```python
from build123d import *

# Parameters (mm, degrees)
F1_R      = 3
F5_DEPTH  = 7
F6_SIZE   = 2
F7_DEPTH  = 15.8
F1_R_2    = 5.35
F8_DEPTH  = 7
F9_SIZE   = 2
F1_R_3    = 7.5
F1_R_4    = 5.05
F10_DEPTH = 3
F1_R_5    = 3.15
F11_DEPTH = 10
F12_DEPTH = 1
F13_DEPTH = 4
F14_W     = 38.3726581931
F14_H     = 0.6922930479
F15_DEPTH = 1


with BuildPart() as f5:
    # F1 (on Top) → F5 (new body)
    with BuildSketch(Plane.XY):
        with BuildLine():
            Line((-67.5440824628, 59.7986807566), (-67.5440824628, 9.7986807566))
            Line((-67.5440824628, 9.7986807566), (-47.5440824628, 9.7986807566))
            Line((-47.5440824628, 9.7986807566), (-47.5440824628, 59.7986807566))
            ThreePointArc((-47.5440824628, 59.7986807566), (-57.5440824628, 69.7986807566), (-67.5440824628, 59.7986807566))
        make_face()
        with Locations((-57.5440824628, 59.7986807566)):
            Circle(F1_R, mode=Mode.SUBTRACT)
    extrude(amount=F5_DEPTH)

    # F6
    f6_edges = [f5.edges().sort_by_distance(p)[0] for p in [
        (-57.544082, 9.798681, 0),
        (-47.544082, 34.798681, 0),
        (-57.544082, 69.798681, 0),
        (-67.544082, 34.798681, 0),
    ]]
    chamfer(f6_edges, length=F6_SIZE)

    # F1 (on Top) → F7 (join)
    with BuildSketch(Plane.XY):
        with Locations((-57.5440824628, 59.7986807566)):
            Circle(F1_R)
    extrude(amount=F7_DEPTH)



with BuildPart() as f8:
    # F1 (on Top) → F8 (new body)
    with BuildSketch(Plane.XY):
        with BuildLine():
            ThreePointArc((-3.5915456533, 60.5911472063), (-13.5915456533, 70.5911472063), (-23.5915456533, 60.5911472063))
            Line((-23.5915456533, 60.5911472063), (-23.5915456533, 10.5911472063))
            Line((-23.5915456533, 10.5911472063), (-3.5915456533, 10.5911472063))
            Line((-3.5915456533, 10.5911472063), (-3.5915456533, 60.5911472063))
        make_face()
        with Locations((-13.5915456533, 60.5911472063)):
            Circle(F1_R_2, mode=Mode.SUBTRACT)
    extrude(amount=F8_DEPTH)

    # F9
    f9_edges = [f8.edges().sort_by_distance(p)[0] for p in [
        (-13.591546, 10.591147, 0),
        (-3.591546, 35.591147, 0),
        (-13.591546, 70.591147, 0),
        (-23.591546, 35.591147, 0),
    ]]
    chamfer(f9_edges, length=F9_SIZE)


with BuildPart() as f10:
    # F1 (on Top) → F10 (new body)
    with BuildSketch(Plane.XY):
        with Locations((-35.6929131355, 62.5116448375)):
            Circle(F1_R_3)
        with Locations((-35.6929131355, 62.5116448375)):
            Circle(F1_R_4, mode=Mode.SUBTRACT)
    extrude(amount=F10_DEPTH)

    # F1 (on Top) → F11 (join)
    with BuildSketch(Plane.XY):
        with Locations((-35.6929131355, 62.5116448375)):
            Circle(F1_R_4)
        with Locations((-35.6929131355, 62.5116448375)):
            Circle(F1_R_5, mode=Mode.SUBTRACT)
    extrude(amount=F11_DEPTH)

    # F1 (on Top) → F12 (join)
    with BuildSketch(Plane.XY):
        with Locations((-35.6929131355, 62.5116448375)):
            Circle(F1_R_5)
    extrude(amount=F12_DEPTH)


with BuildPart() as f13:
    # F1 (on Top) → F13 (new body)
    with BuildSketch(Plane.XY):
        with BuildLine():
            Line((-69.5440824628, 59.7986807566), (-69.5440824628, 7.7986807566))
            Line((-69.5440824628, 7.7986807566), (-45.5440824628, 7.7986807566))
            Line((-45.5440824628, 7.7986807566), (-45.5440824628, 59.7986807566))
            ThreePointArc((-45.5440824628, 59.7986807566), (-57.5440824628, 71.7986807566), (-69.5440824628, 59.7986807566))
        make_face()
        with BuildLine():
            ThreePointArc((-68.5440824628, 59.7986807566), (-57.5440824628, 70.7986807566), (-46.5440824628, 59.7986807566))
            Line((-46.5440824628, 59.7986807566), (-46.5440824628, 8.7986807566))
            Line((-46.5440824628, 8.7986807566), (-68.5440824628, 8.7986807566))
            Line((-68.5440824628, 8.7986807566), (-68.5440824628, 59.7986807566))
        make_face(mode=Mode.SUBTRACT)
    extrude(amount=F13_DEPTH)


with BuildPart() as f13b:
    # F1 (on Top) → F13, piece 2 (new body)
    with BuildSketch(Plane.XY):
        with BuildLine():
            Line((-25.5915456533, 60.5911472063), (-25.5915456533, 8.5911472063))
            Line((-25.5915456533, 8.5911472063), (-1.5915456533, 8.5911472063))
            Line((-1.5915456533, 8.5911472063), (-1.5915456533, 60.5911472063))
            ThreePointArc((-1.5915456533, 60.5911472063), (-13.5915456533, 72.5911472063), (-25.5915456533, 60.5911472063))
        make_face()
        with BuildLine():
            Line((-2.5915456533, 9.5911472063), (-24.5915456533, 9.5911472063))
            Line((-24.5915456533, 9.5911472063), (-24.5915456533, 60.5911472063))
            ThreePointArc((-24.5915456533, 60.5911472063), (-13.5915456533, 71.5911472063), (-2.5915456533, 60.5911472063))
            Line((-2.5915456533, 60.5911472063), (-2.5915456533, 9.5911472063))
        make_face(mode=Mode.SUBTRACT)
    extrude(amount=F13_DEPTH)


with BuildPart() as f5_1:
    add(f5.part)

    add(f8.part)  # F15 merges F8

    add(f10.part)  # F15 merges F10

    add(f13.part)  # F15 merges F13

    add(f13b.part)  # F15 merges F13b
    # F14 (on Top) → F15 (join)
    with BuildSketch(Plane.XY):
        with Locations((-36.1423902214, 55.9608265758)):
            Rectangle(F14_W, F14_H)
    extrude(amount=F15_DEPTH)


solid = f5_1.part
```
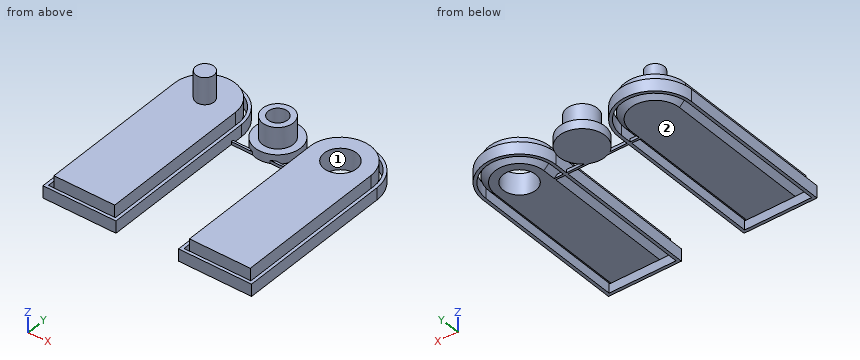
Here's how the part is built. I have some questions about the finished solid (model axes, mm). Face numbers are marked on the shaded views. Round coordinates to 2 decimals unless told otherwise and drop trailing zeros. Loops run counter-clockwise (first coordinate to the right, second up) from the corner with the lowest first, then second, coordinate; pieces in that order, holes last.
1. Suppose I cut it at B-B, the plane x = -58.5. Give the number of separate pieces and of enclosed holes in the cut face, and give its area (3 significant figures).
Answers:
separate pieces: 3
enclosed holes: 0
area: 474 mm2
2. If I drill on probe 1 along X at (y, z) = (34, 5.75); probe 2 along X at (y, z) = (48.5, 1.75); probe 3 along X at (y, z) = (38.5, 2.75), over which ranges is the centre line in solid material (lowest first)?
Answers:
probe 1: x = -67.54 to -47.54, -23.59 to -3.59
probe 2: x = -69.54 to -68.54, -67.29 to -47.79, -46.54 to -45.54, -25.59 to -24.59, -23.34 to -3.84, -2.59 to -1.59
probe 3: x = -69.54 to -68.54, -67.54 to -47.54, -46.54 to -45.54, -25.59 to -24.59, -23.59 to -3.59, -2.59 to -1.59
3. Suppose I cut it at A-A, the plane y = 30.5. Please give me the cut outline in (x, z).
Answers:
outline: (-69.54, 0) - (-68.54, 0) - (-68.54, 4) - (-69.54, 4) - close; (-67.54, 2) - (-65.54, 0) - (-49.54, 0) - (-47.54, 2) - (-47.54, 7) - (-67.54, 7) - close; (-46.54, 0) - (-45.54, 0) - (-45.54, 4) - (-46.54, 4) - close; (-25.59, 0) - (-24.59, 0) - (-24.59, 4) - (-25.59, 4) - close; (-23.59, 2) - (-21.59, 0) - (-5.59, 0) - (-3.59, 2) - (-3.59, 7) - (-23.59, 7) - close; (-2.59, 0) - (-1.59, 0) - (-1.59, 4) - (-2.59, 4) - close
4. Thinking about a two-plate mould opening in X: for the marked faces 1 and 2, which applies, released by +X, released by -X, zero draft, split by the parting line, or undercut?
Answers:
face 1: undercut
face 2: zero draft
5. Suppose I cut it at C-C, the plane z = 14.5. Please give me the cut outline in (x, y).
Answers:
outline: circle Ø6 at (-57.54, 59.8)
6. Will these pins go through, and if not, where does the flat tip stop? pin 1 (12 mm diameter, centred on x = -55.5, y = 47, fed in from +Z); pin 2 (5 mm diameter, centred on x = -35, y = 61, fed in from +Z); pin 3 (4.5 mm diameter, centred on x = -11, z = 2.5, fed in from +Y).
Answers:
pin 1: stops at z = 7
pin 2: stops at z = 10
pin 3: stops at y = 72.59
